Autodesk Fusion 360 part; units mm, degrees
sketch "Sketch1" plane through (0, 0, 0) normal (0, 1, 0) x (1, 0, 0)
  line L0 (-107.4349, 34.7679) -> (245.6251, 34.7679)
  line L1 (245.6251, 34.7679) -> (245.6251, -118.2321)
  line L2 (245.6251, -118.2321) -> (-107.4349, -118.2321)
  line L3 (-107.4349, -118.2321) -> (-107.4349, 34.7679)
  line L4 (-107.4349, 34.7679) -> (245.6251, 34.7679)
  line L5 (245.6251, 34.7679) -> (245.6251, 29.7679)
  line L6 (-107.4349, 29.7679) -> (-107.4349, 34.7679)
  line L7 (245.6251, 34.7679) -> (240.6251, 34.7679)
  line L8 (157.6216, -118.2321) -> (245.6251, -118.2321)
  line L9 (245.6251, -118.2321) -> (245.6251, 34.7679)
  line L10 (245.6251, -118.2321) -> (-107.4349, -118.2321)
  line L11 (-107.4349, -118.2321) -> (-107.4349, -113.2321)
  line L12 (245.6251, -113.2321) -> (245.6251, -118.2321)
  line L13 (-107.4349, -118.2321) -> (-30.4984, -118.2321)
  line L14 (-102.4349, 34.7679) -> (-107.4349, 34.7679)
  line L15 (-107.4349, 34.7679) -> (-107.4349, -118.2321)
  line L16 (-107.4349, -118.2321) -> (-24.9576, -118.2321)
  line L17 (-96.894, -113.2321) -> (-96.894, -107.2397)
  line L18 (-96.894, -107.2397) -> (-102.4349, -107.2397)
  line L19 (-107.4349, -107.2397) -> (-107.4349, -118.2321)
  circle A0 centre (-103.1349, -114.3777) radius 2.1
  line L20 (-106.1349, -119.3752) -> (-99.8349, -119.3752)
  line L21 (69.0951, -118.2321) -> (69.0951, 34.7679) construction
  line L22 (245.6251, -41.7321) -> (-107.4349, -41.7321) construction
  line L23 (235.0843, -113.2321) -> (235.0843, -107.2397)
  line L24 (235.0843, -107.2397) -> (240.6251, -107.2397)
  circle A1 centre (241.3251, -114.3777) radius 2.1
  line L25 (-96.894, -113.2321) -> (235.0843, -113.2321)
  circle A2 centre (-103.1349, 30.9136) radius 2.1
  line L26 (-96.894, 29.7679) -> (-96.894, 23.7756)
  line L27 (-96.894, 23.7756) -> (-102.4349, 23.7756)
  line L28 (235.0843, 23.7756) -> (240.6251, 23.7756)
  line L29 (235.0843, 29.7679) -> (235.0843, 23.7756)
  circle A3 centre (241.3251, 30.9136) radius 2.1
  line L30 (240.6251, 23.7756) -> (240.6251, -107.2397)
  line L31 (235.0843, 29.7679) -> (-96.894, 29.7679)
  line L32 (-102.4349, -107.2397) -> (-102.4349, 23.7756)
  dimension "d1" = 153
  dimension "d2" = 353.06
  dimension "d3" = 5
  dimension "d4" = 5
  dimension "d5" = 5
  dimension "d6" = 5
  dimension "d8" = 4.2
  dimension "d9" = 4.3
  dimension "d10" = 6.3
  dimension "d11" = 1.3
  dimension "d14" = 3.8543
  dimension "d15" = 10.5408
  dimension "d16" = 10.9923
  dimension "d17" = 5
  dimension "d18" = 5
  dimension "d19" = 5
extrude "Extrude1" add sketch "Sketch1" along normal blind 11.43
extrude "Extrude2" add 1 faces at (216.2906, 3.81, 118.2321) along direction (0, 0, 1) blind 5.08
extrude "Extrude3" add 1 faces at (127.9385, 7.62, -34.7679) along direction (0, 0, -1) blind 5.08
equation "d9 = 1.8 mm + 2.5 mm"
For this review, take the finished solid that the model builds, in its own axes (mm). A direction names the side the tool comes from. Round coordinates to 2 decimals unless told otherwise and drop trailing zeros. Write each loop counter-clockwise with the first axis right and the second up, starting at its lowest first coordinate (ties: lowest second). Pieces come first, ordered by that corner, then holes. Notation, with made-up numbers: (7, 89) - (43, 89) arc R23 cw to (43, 101) - close; hole circle Ø11 at (-21, -5.5). An arc over 180 degrees is marked (long way). Write each question's results on one line, items separated by ' | '.
Item 1: To check wall thickness, follow line 1 along Z through (x, y) = (205, 1.25); line 2 along X through (y, z) = (6.75, 14); line 3 along Z through (x, y) = (32.5, 6.75). State the ranges of each line that lie inside material, in increasing order. Write a range as from..to.
Calculated:
line 1: z = -39.85..-29.77, 113.23..123.31 | line 2: x = -107.43..-102.43, 240.63..245.63 | line 3: z = -39.85..-29.77, 113.23..118.23
Item 2: For faces 1 (the face through (27, 6, 118.232)), 2 (the face through (81, 11.43, -30)), 3 (the face through (235.084, 6, -27)), list the 3-axis set-ups (+Z, -Z, +X, -X, +Y, -Y) from which the entire face can be reached by the end or side of a thin tool; tool diameter is ignored.
Calculated:
face 1: +Z, -X, +Y, -Y | face 2: +Z, -Z, +X, -X, +Y | face 3: +Y, -Y
Item 3: Draft analysis for pull direction X (two halves, no side actions). For faces 4 (the face through (-102.435, 6, 43)), 5 (the face through (245.625, 6, 43)), 6 (the face through (67, 6, -39.848)), state which applies: pulls with the +X half, pulls with the -X half, needs draft (parallel to the pull), parting line crosses it, or undercut.
Calculated:
face 4: undercut | face 5: pulls with the +X half | face 6: needs draft
Item 4: Take a section at B-B on z = 67.5. State the section outline as (x, y) points, then the cut area to 3 significant figures.
Calculated:
outline: (-107.43, 0) - (-102.43, 0) - (-102.43, 11.43) - (-107.43, 11.43) - close; (240.63, 0) - (245.63, 0) - (245.63, 11.43) - (240.63, 11.43) - close | area: 114 mm^2
Item 5: For pin 1 (3.5 mm diameter, centred on x = 36, y = 5.5, fed in from +Z), flat-tipped, find the tip position at first contact; note if it passes through.
Calculated:
pin 1: stops at z = 118.23
Item 6: Take a section at C-C on y = 3.5. State the section outline as (x, z) points, then the cut area to 3 significant figures.
Calculated:
outline: (-107.43, -39.85) - (245.63, -39.85) - (245.63, 123.31) - (157.62, 123.31) - (157.62, 118.23) - (-107.43, 118.23) - close; hole circle Ø4.2 at (-103.13, -30.91); hole circle Ø4.2 at (-103.13, 114.38); hole (-102.43, -23.78) - (-96.89, -23.78) - (-96.89, -29.77) - (235.08, -29.77) - (235.08, -23.78) - (240.63, -23.78) - (240.63, 107.24) - (235.08, 107.24) - (235.08, 113.23) - (-96.89, 113.23) - (-96.89, 107.24) - (-102.43, 107.24) - close; hole circle Ø4.2 at (241.33, -30.91); hole circle Ø4.2 at (241.33, 114.38) | area: 7,280 mm^2
Item 7: Take a section at A-A on x = -33.5. State the section outline as (y, z) points, then the cut area to 3 significant figures.
Calculated:
outline: (0, -39.85) - (11.43, -39.85) - (11.43, -29.77) - (0, -29.77) - close; (0, 113.23) - (11.43, 113.23) - (11.43, 118.23) - (0, 118.23) - close | area: 172 mm^2
